The listing builds one solid part. Answer for the finished solid, in the listing's coordinates (mm). Face numbers are marked on the shaded views. A direction names the side the tool comes from. Coordinates: 2 decimals unless noted, no trailing zeros. Order: outer loops, then holes, each group sorted by start corner. A loop starts at its lowest first (then second) coordinate and runs counter-clockwise, first axis right, second up. Notation, with made-up numbers: (-39, -26) -> (-15, -26) arc R7 ccw to (-15, -15) -> close; hole circle Ø4 at (76, 32.5). An arc over 180 degrees is marked (long way). Return JSON: item names as keys, results as strings.
```python
from build123d import *

# Parameters (mm, degrees)
F0_W     = 100
F0_H     = 100
F1_DEPTH = 60
F5_DEPTH = 90


with BuildPart() as f1:
    # F0 (on Top) → F1 (new body)
    with BuildSketch(Plane.XY):
        with Locations((-50, 50)):
            Rectangle(F0_W, F0_H)
    extrude(amount=F1_DEPTH)

    # F4 (on offset) → F5 (cut)
    with BuildSketch(Plane(origin=(0, 95, 0), x_dir=(-1, 0, 0), z_dir=(0, 1, 0))):
        Polygon((49.9035641551, 59.3563504517), (4.9081675543, 0), (94.8989607559, 0), align=None)
    extrude(amount=-F5_DEPTH, mode=Mode.SUBTRACT)


solid = f1.part
```
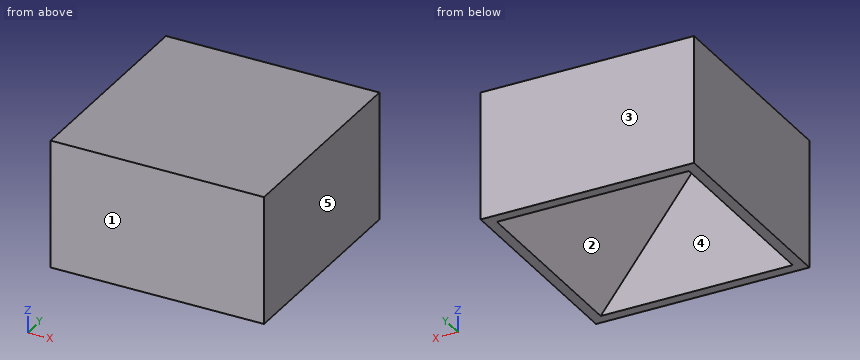
Item 1: The part is cut by section A-A on z = 43. Determine the outline of the cut face in (x, y).
Answer list:
{"outline": "(-100, 0) -> (0, 0) -> (0, 100) -> (-100, 100) -> close; hole (-62.3, 5) -> (-37.5, 5) -> (-37.5, 95) -> (-62.3, 95) -> close"}
Item 2: The part is cut by section D-D on z = 17. Determine the outline of the cut face in (x, y).
Answer list:
{"outline": "(-100, 0) -> (0, 0) -> (0, 100) -> (-100, 100) -> close; hole (-82.01, 5) -> (-17.8, 5) -> (-17.8, 95) -> (-82.01, 95) -> close"}
Item 3: The part is cut by section B-B on y = 89. Determine the outline of the cut face in (x, z).
Answer list:
{"outline": "(-100, 0) -> (-94.9, 0) -> (-49.9, 59.36) -> (-4.91, 0) -> (0, 0) -> (0, 60) -> (-100, 60) -> close"}
Item 4: Flat-ended cylindrical pins translate along their axes: pin 1 (3 mm diameter, centred on x = -85, z = 43.5, fed in from -Y); pin 2 (5 mm diameter, centred on x = -47.5, y = 60.5, fed in from -Z). Find the tip coordinate at first contact, or state that the pin passes through.
Answer list:
{"pin 1": "y = 0", "pin 2": "z = 52.89"}
Item 5: Find the intervals of material crossed by probe 1 along Y at (x, z) = (-47, 10); probe 2 along X at (y, z) = (36.5, 52); probe 3 along X at (y, z) = (88, 34.5), in increasing order.
Answer list:
{"probe 1": "0 to 5, 95 to 100", "probe 2": "-100 to -55.48, -44.33 to 0", "probe 3": "-100 to -68.75, -31.06 to 0"}
Item 6: Determine the mould class of the marked faces 3, 4 and 5 for opening direction X: pulls with the +X half, pulls with the -X half, needs draft (parallel to the pull), parting line crosses it, or undercut.
Answer list:
{"face 3": "needs draft", "face 4": "undercut", "face 5": "pulls with the +X half"}
Item 7: The part is cut by section C-C on x = -37.5. Determine the outline of the cut face in (y, z), plus the area to 3 significant figures.
Answer list:
{"outline": "(0, 0) -> (5, 0) -> (5, 42.99) -> (95, 42.99) -> (95, 0) -> (100, 0) -> (100, 60) -> (0, 60) -> close", "area": "2,130 mm2"}
Item 8: Which of the six approach directions +Z, -Z, +X, -X, +Y, -Y give full straight-line access (tool end or side, diameter ignored) to the marked faces 1 and 2?
Answer list:
{"face 1": "+Z, -Z, +X, -X, -Y", "face 2": "-Z"}
